```python
from build123d import *

# Parameters (mm, degrees)
SKETCH_1_R               = 47.75
EXTRUDE_1_DEPTH          = 14
SKETCH_2_R               = 9.65
EXTRUDE_2_DEPTH          = 8.4
SKETCH_3_R               = 5
CUT_EXTRUDE_1_DEPTH      = 22.4
CUT_EXTRUDE_2_REACH      = 73.147
CUT_EXTRUDE_2_END_RADIUS = 9.65
SKETCH_6_R               = 2
CUT_EXTRUDE_START        = -2
SKETCH_7_R               = 39
SKETCH_7_R_2             = 9.65
CUT_EXTRUDE_3_DEPTH      = 2
SKETCH_8_R               = 39
SKETCH_8_R_2             = 9.65
CUT_EXTRUDE_4_DEPTH      = 2
CUT_EXTRUDE_5_REACH      = 70.587
SKETCH_9_R               = 7.5


with BuildPart() as part:
    # 草图1 → 凸台-拉伸1 (new body)
    with BuildSketch(Plane.XY):
        Circle(SKETCH_1_R)
    extrude(amount=EXTRUDE_1_DEPTH)

    # 草图2 → 凸台-拉伸2 (add)
    with BuildSketch(Plane.XY.offset(14)):
        Circle(SKETCH_2_R)
    extrude(amount=EXTRUDE_2_DEPTH)

    # 草图3 → 切除-拉伸1 (cut)
    with BuildSketch(Plane.XY.offset(22.4)):
        Circle(SKETCH_3_R)
    extrude(amount=-CUT_EXTRUDE_1_DEPTH, mode=Mode.SUBTRACT)

    # 切除-拉伸2: up to this cylinder (the profile starts inside it)
    cut_extrude_2_end = Plane(origin=(0, 0, 19.2), z_dir=(0, 0, -1)) * Cylinder(CUT_EXTRUDE_2_END_RADIUS, 166.594, mode=Mode.PRIVATE)
    # 草图6 → 切除-拉伸2 (cut, up to the surface)
    with BuildSketch(Plane(origin=(0, 0, 0), x_dir=(0, 0, -1), z_dir=(1, 0, 0)), mode=Mode.PRIVATE) as cut_extrude_2_sk1:
        with Locations((-19.2, 0)):
            Circle(SKETCH_6_R)
    cut_extrude_2_tool1 = extrude(cut_extrude_2_sk1.sketch, amount=-CUT_EXTRUDE_2_REACH, mode=Mode.PRIVATE) & cut_extrude_2_end
    add(cut_extrude_2_tool1.solids().sort_by_distance((0, 0, 19.2))[0], mode=Mode.SUBTRACT)

    # 草图7 → 切除-拉伸3 (cut)
    with BuildSketch(Plane.XY.offset(14).offset(CUT_EXTRUDE_START)):
        Circle(SKETCH_7_R)
        Circle(SKETCH_7_R_2, mode=Mode.SUBTRACT)
    extrude(amount=CUT_EXTRUDE_3_DEPTH, mode=Mode.SUBTRACT)

    # 草图8 → 切除-拉伸4 (cut)
    with BuildSketch(Plane(origin=(0, 0, 0), x_dir=(-1, 0, 0), z_dir=(0, 0, -1))):
        with Locations(Location((0, 0, 0), (0, 0, 180))):
            Circle(SKETCH_8_R)
        with Locations(Location((0, 0, 0), (0, 0, 180))):
            Circle(SKETCH_8_R_2, mode=Mode.SUBTRACT)
    extrude(amount=-CUT_EXTRUDE_4_DEPTH, mode=Mode.SUBTRACT)

    # 草图9 → 切除-拉伸5 (cut, up to next)
    with BuildSketch(Plane.XY.offset(12), mode=Mode.PRIVATE) as cut_extrude_5_sk1:
        with Locations((0, 24)):
            Circle(SKETCH_9_R)
    cut_extrude_5_tool1 = extrude(cut_extrude_5_sk1.sketch, amount=-CUT_EXTRUDE_5_REACH, mode=Mode.PRIVATE) & part.part
    # 草图9 → 切除-拉伸5 (cut, up to next)
    with BuildSketch(Plane.XY.offset(12), mode=Mode.PRIVATE) as cut_extrude_5_sk2:
        with Locations((22.825356391, 7.416407865)):
            Circle(SKETCH_9_R)
    cut_extrude_5_tool2 = extrude(cut_extrude_5_sk2.sketch, amount=-CUT_EXTRUDE_5_REACH, mode=Mode.PRIVATE) & part.part
    # 草图9 → 切除-拉伸5 (cut, up to next)
    with BuildSketch(Plane.XY.offset(12), mode=Mode.PRIVATE) as cut_extrude_5_sk3:
        with Locations((14.106846055, -19.416407865)):
            Circle(SKETCH_9_R)
    cut_extrude_5_tool3 = extrude(cut_extrude_5_sk3.sketch, amount=-CUT_EXTRUDE_5_REACH, mode=Mode.PRIVATE) & part.part
    # 草图9 → 切除-拉伸5 (cut, up to next)
    with BuildSketch(Plane.XY.offset(12), mode=Mode.PRIVATE) as cut_extrude_5_sk4:
        with Locations((-14.106846055, -19.416407865)):
            Circle(SKETCH_9_R)
    cut_extrude_5_tool4 = extrude(cut_extrude_5_sk4.sketch, amount=-CUT_EXTRUDE_5_REACH, mode=Mode.PRIVATE) & part.part
    # 草图9 → 切除-拉伸5 (cut, up to next)
    with BuildSketch(Plane.XY.offset(12), mode=Mode.PRIVATE) as cut_extrude_5_sk5:
        with Locations((-22.825356391, 7.416407865)):
            Circle(SKETCH_9_R)
    cut_extrude_5_tool5 = extrude(cut_extrude_5_sk5.sketch, amount=-CUT_EXTRUDE_5_REACH, mode=Mode.PRIVATE) & part.part
    add(cut_extrude_5_tool1.solids().sort_by_distance((0, 24, 12))[0], mode=Mode.SUBTRACT)
    add(cut_extrude_5_tool2.solids().sort_by_distance((22.825356, 7.416408, 12))[0], mode=Mode.SUBTRACT)
    add(cut_extrude_5_tool3.solids().sort_by_distance((14.106846, -19.416408, 12))[0], mode=Mode.SUBTRACT)
    add(cut_extrude_5_tool4.solids().sort_by_distance((-14.106846, -19.416408, 12))[0], mode=Mode.SUBTRACT)
    add(cut_extrude_5_tool5.solids().sort_by_distance((-22.825356, 7.416408, 12))[0], mode=Mode.SUBTRACT)


solid = part.part
```
Could you check a few things on this model? Use its own coordinates, in mm. A direction names the side the tool comes from. Coordinates: 2 decimals unless noted, no trailing zeros. Loops run counter-clockwise (first coordinate to the right, second up) from the corner with the lowest first, then second, coordinate; pieces in that order, holes last. Notation, with made-up numbers: M 51.5,35.25 L 70.5,35.25 A28 ccw 70.5,74.25 Z; hole C 73,11.25 d7. An arc over 180 degrees is marked long. Put each result on its own line as item: value. Start each with the question number.
(1) Suppose I cut it at D-D on z = 7.5. Please give me the cut outline in (x, y), then the cut area to 3 significant figures.
(2) Will these pins go through, and if not, where does the flat tip stop? P1, Ø1.5, axis at y = 30, z = 8, coming from the -X side; P2, Ø24, axis at x = -14.11, y = -19.42, coming from the -Z side; P3, Ø1, axis at x = 8.5, z = 7.5, coming from the -Y side.
(3) For faces 4 (the face through (-7.081, 1.983, 19.46)), 5 (the face through (-5.077, 38.668, 12.986)), 6 (the face through (9.204, -2.899, 0.986)), which set-ups out of +Z, -Z, +X, -X, +Y, -Y let a thin tool reach every point of the face, with its end or its side?
(4) Suppose I cut it at C-C on y = 24. Please give me the cut outline in (x, z), then the cut area to 3 significant figures.
(5) Suppose I cut it at A-A on x = 0. Please give me the cut outline in (y, z), then the cut area to 3 significant figures.
(6) Suppose I cut it at B-B on x = -23. Please give me the cut outline in (y, z).
(7) I need wall thicknesses on line 1 (Y direction, x = 0, z = 9.75); line 2 (Y direction, x = 0, z = 13.15); line 3 (Z direction, x = 28.5, y = 19.5). Which ranges of each line are inside material? Lowest first, please. Write a range as from..to.
(8) Thinking about a two-plate mould opening in Y: for faces 1 (the face through (-10.351, -46.615, 6.902)), 2 (the face through (4, -4, 0)), 3 (the face through (8, -8, 12)), which applies, pulls with the +Y half, pulls with the -Y half, needs draft (parallel to the pull), parting line crosses it, or undercut?
Solutions:
1. outline: C 0,0 d95.5; hole C -22.83,7.42 d15; hole C -14.11,-19.42 d15; hole C 0,24 d15; hole C 0,0 d10; hole C 14.11,-19.42 d15; hole C 22.83,7.42 d15
1. area: 6,200 mm2
2. P1: stops at x = -37.74
2. P2: stops at z = 2
2. P3: stops at y = -47.08
3. face 4: -X
3. face 5: +Z
3. face 6: -Z
4. outline: M -41.28,0 L -30.74,0 L -30.74,2 L -7.5,2 L -7.5,12 L -30.74,12 L -30.74,14 L -41.28,14 Z; M 7.5,2 L 30.74,2 L 30.74,0 L 41.28,0 L 41.28,14 L 30.74,14 L 30.74,12 L 7.5,12 Z
4. area: 760 mm2
5. outline: M -47.75,0 L -39,0 L -39,2 L -9.65,2 L -9.65,0 L -5,0 L -5,22.4 L -9.65,22.4 L -9.65,12 L -39,12 L -39,14 L -47.75,14 Z; M 5,0 L 9.65,0 L 9.65,2 L 16.5,2 L 16.5,12 L 9.65,12 L 9.65,22.4 L 5,22.4 Z; M 31.5,2 L 39,2 L 39,0 L 47.75,0 L 47.75,14 L 39,14 L 39,12 L 31.5,12 Z
5. area: 890 mm2
6. outline: M -41.85,0 L -31.5,0 L -31.5,2 L -0.08,2 L -0.08,12 L -31.5,12 L -31.5,14 L -41.85,14 Z; M 14.91,2 L 31.5,2 L 31.5,0 L 41.85,0 L 41.85,14 L 31.5,14 L 31.5,12 L 14.91,12 Z
7. line 1: y = -47.75..-5, 5..16.5, 31.5..47.75
7. line 2: y = -47.75..-39, -9.65..-5, 5..9.65, 39..47.75
7. line 3: z = 2..12
8. face 1: parting line crosses it
8. face 2: needs draft
8. face 3: undercut
